Source: CAD feature listing. Evaluate the final solid. Frame: model axes, mm. A direction names the side the tool comes from. Coordinates: 2 decimals unless noted, no trailing zeros. Write each loop counter-clockwise with the first axis right and the second up, starting at its lowest first coordinate (ties: lowest second). Pieces come first, ordered by that corner, then holes. Notation, with made-up numbers: (68, 37.5) - (90, 37.5) arc R7 ccw to (90, 46.5) - close; hole circle Ø4 at (61.25, -19.75). An arc over 180 degrees is marked (long way). One line per question, with ' | ' between items. Start each with the question number.
Q1. Access query for faces 1 (the face through (2.71, -7.95, 20.46)), 2 (the face through (27.035, -3.042, -12.8)), 3 (the face through (0, -10, -26)), 4 (the face through (1.802, -15.437, 5.723)). Directions: +Z, -Z, +X, -X, +Y, -Y. A direction counts if a zero-diameter tool reaches every point of the face in a straight line with its end or side. Return the directions, or none.
Q2. Cut plane D-D, the plane y = -3.5. Return loops of the section in (x, z), plus the area to 3 significant figures.
Q3. Cut plane A-A, the plane y = -15. Return loops of the section in (x, z), plus the area to 3 significant figures.
Q4. Cut plane B-B, the plane z = 0. Return loops of the section in (x, y).
Q5. Cut plane C-C, the plane x = 13.5. Return loops of the section in (y, z), plus the area to 3 significant figures.
Q6. Line query: line 1 (X direction, y = -7.15, z = 0); line 2 (Z direction, x = 3.45, y = -15); line 3 (Z direction, x = 2.2, y = -15). Output: solid intervals per line, ascending.
Q7. Draft query along Y for faces 5 (the face through (2.71, -7.92, -20.64)), 6 (the face through (22.445, -7.507, 0.846)), 7 (the face through (21, 0, -1)), 8 (the face through (8, -20, 0)). Return one class per face: +Y half, -Y half, draft (parallel to the pull), parting line (faces both ways), or undercut.
Q8. Contact query for flat-ended pins moving along their axis: P1, Ø1.5, axis at y = -12, z = 23, coming from the +X side; P2, Ø14.5, axis at x = 16.5, z = -1, coming from the -Y side; P3, Ø6, axis at x = 24, y = -5.5, coming from the -Z side; P4, Ø4, axis at x = 6, z = 22.5, coming from the +Y side. Output: stop coordinate, or through.
```python
from build123d import *

# Parameters (mm, degrees)
SKETCH_1_R          = 6
EXTRUDE_1_DEPTH     = 20
SKETCH_2_R          = 6.1
EXTRUDE_2_DEPTH     = 11
SKETCH_3_R          = 3.4
CUT_EXTRUDE_1_DEPTH = 60.989832472
SKETCH_4_R          = 2.1
CUT_EXTRUDE_2_DEPTH = 10
CUT_EXTRUDE_3_DEPTH = 63.271823484
CUT_EXTRUDE_4_DEPTH = 12
SKETCH_7_R          = 6.5
CUT_EXTRUDE_5_DEPTH = 1
SKETCH_8_R          = 4
CUT_EXTRUDE_6_DEPTH = 60.554848669
CUT_EXTRUDE_7_DEPTH = 60.344586948
CUT_EXTRUDE_8_DEPTH = 2
CHAMFER_1_SIZE      = 0.2


with BuildPart() as part:
    # 草图1 → 凸台-拉伸1 (new body)
    with BuildSketch(Plane(origin=(0, 0, 0), x_dir=(1, 0, 0), z_dir=(0, 1, 0))):
        with BuildLine():
            Line((0, 41.7), (0, 10.918333206))
            ThreePointArc((0, 10.918333206), (-0.463653568, 9.637849063), (-1.63963964, 8.951065962))
            ThreePointArc((-1.63963964, 8.951065962), (-9.1, 0), (-1.63963964, -8.951065962))
            ThreePointArc((-1.63963964, -8.951065962), (-0.463653568, -9.637849063), (0, -10.918333206))
            Line((0, -10.918333206), (0, -41.7))
            ThreePointArc((0, -41.7), (41.7, 0), (0, 41.7))
        make_face()
        with Locations(Location((0, 0, 0), (0, 0, 270))):
            Circle(SKETCH_1_R, mode=Mode.SUBTRACT)
    extrude(amount=EXTRUDE_1_DEPTH)

    # 草图2 → 凸台-拉伸2 (add)
    with BuildSketch(Plane.XZ):
        Circle(SKETCH_2_R)
    extrude(amount=-EXTRUDE_2_DEPTH)

    # 草图3 → 切除-拉伸1 (cut, through all)
    with BuildSketch(Plane(origin=(0, 11, 0), x_dir=(1, 0, 0), z_dir=(0, 1, 0))):
        with Locations(Location((0, 0, 0), (0, 0, 270))):
            Circle(SKETCH_3_R)
    extrude(amount=-CUT_EXTRUDE_1_DEPTH, mode=Mode.SUBTRACT)

    # 草图4 → 切除-拉伸2 (cut)
    with BuildSketch(Plane.ZY):
        with Locations((33.667083302, 15)):
            Circle(SKETCH_4_R)
        with Locations((20.918333206, 10)):
            Circle(SKETCH_4_R)
        with Locations(Location((-33.667083302, 15, 0), (0, 0, 180))):
            Circle(SKETCH_4_R)
        with Locations(Location((-20.918333206, 10, 0), (0, 0, 180))):
            Circle(SKETCH_4_R)
    extrude(amount=-CUT_EXTRUDE_2_DEPTH, mode=Mode.SUBTRACT)


with BuildPart() as body_2:
    # 镜向1: mirrored copy
    add(part.part.mirror(Plane.ZX))

    # 草图5 → 切除-拉伸3 (cut, through all)
    with BuildSketch(Plane(origin=(0, 0, 0), x_dir=(1, 0, 0), z_dir=(0, 1, 0))):
        with BuildLine():
            Line((40.483206395, 10), (40.483206395, -10))
            ThreePointArc((40.483206395, -10), (41.394683878, -5.036878663), (41.7, 0))
            ThreePointArc((41.7, 0), (41.394683878, 5.036878663), (40.483206395, 10))
        make_face()
    extrude(amount=-CUT_EXTRUDE_3_DEPTH, mode=Mode.SUBTRACT)

    # 草图6 → 切除-拉伸4 (cut)
    with BuildSketch(Plane.XZ.offset(20)):
        with BuildLine():
            Line((6, -36.124783736), (6, -6.841783393))
            ThreePointArc((6, -6.841783393), (9.1, 0), (6, 6.841783393))
            Line((6, 6.841783393), (6, 36.124783736))
            ThreePointArc((6, 36.124783736), (6.747974614, 37.684409471), (8.432432432, 38.077474749))
            ThreePointArc((8.432432432, 38.077474749), (39, 0), (8.432432432, -38.077474749))
            ThreePointArc((8.432432432, -38.077474749), (6.747974614, -37.684409471), (6, -36.124783736))
        make_face()
    extrude(amount=-CUT_EXTRUDE_4_DEPTH, mode=Mode.SUBTRACT)

    # 草图7 → 切除-拉伸5 (cut)
    with BuildSketch(Plane.XZ.offset(8)):
        with Locations(Location((16, 0, 0), (0, 0, 270))):
            Circle(SKETCH_7_R)
    extrude(amount=-CUT_EXTRUDE_5_DEPTH, mode=Mode.SUBTRACT)

    # 草图8 → 切除-拉伸6 (cut, through all)
    with BuildSketch(Plane.XZ.offset(7)):
        with Locations(Location((16, 0, 0), (0, 0, 270))):
            Circle(SKETCH_8_R)
    extrude(amount=-CUT_EXTRUDE_6_DEPTH, mode=Mode.SUBTRACT)

    # 草图9 → 切除-拉伸7 (cut, through all)
    with BuildSketch(Plane.XZ.offset(8)):
        with BuildLine():
            ThreePointArc((22.891243611, -20.998113284), (30.339314214, -16.81648203), (35.645345475, -10.122766478))
            ThreePointArc((35.645345475, -10.122766478), (34.525042064, -6.62063566), (31.022911246, -7.740939071))
            ThreePointArc((31.022911246, -7.740939071), (26.965357928, -12.859662729), (21.269774526, -16.057380747))
            ThreePointArc((21.269774526, -16.057380747), (19.6101428, -19.338481558), (22.891243611, -20.998113284))
        make_face()
    extrude(amount=-CUT_EXTRUDE_7_DEPTH, mode=Mode.SUBTRACT)

    # 草图10 → 切除-拉伸8 (cut)
    with BuildSketch(Plane.XZ.offset(8)):
        with BuildLine():
            ThreePointArc((23.712726546, -22.721297552), (31.438040853, -18.105017627), (37.217069697, -11.206224463))
            ThreePointArc((37.217069697, -11.206224463), (35.608500049, -5.048911438), (29.451187024, -6.657481086))
            ThreePointArc((29.451187024, -6.657481086), (25.598501128, -11.256676528), (20.44829159, -14.334196479))
            ThreePointArc((20.44829159, -14.334196479), (17.886958532, -20.159964494), (23.712726546, -22.721297552))
        make_face()
    extrude(amount=-CUT_EXTRUDE_8_DEPTH, mode=Mode.SUBTRACT)

    # 倒角1
    chamfer_1_edges = [body_2.edges().sort_by_distance(p)[0] for p in [
        (0, -10, 41.7),
        (0, -10, -41.7),
    ]]
    chamfer(chamfer_1_edges, length=CHAMFER_1_SIZE)


solid = body_2.part
```
Reply:
1) face 1: -X | face 2: +Y, -Y | face 3: -Z, -X, +Y, -Y | face 4: -Y
2) outline: (-1.64, -8.95) arc R2 cw to (0, -10.92) - (0, -41.5) - (0.2, -41.7) arc R41.7 ccw to (40.48, -10) - (40.48, 10) arc R41.7 ccw to (0.2, 41.7) - (0, 41.5) - (0, 10.92) arc R2 cw to (-1.64, 8.95) arc R9.1 ccw to start; hole circle Ø6.8 at (0, 0); hole circle Ø8 at (16, 0); hole (21.27, -16.06) arc R2.6 ccw to (22.89, -21) arc R22.1 ccw to (35.65, -10.12) arc R2.6 ccw to (31.02, -7.74) arc R16.9 cw to start | area: 2,660 mm^2
3) outline: (-1.64, -8.95) arc R2 cw to (0, -10.92) - (0, -31.57) - (6, -31.57) - (6, -6.84) arc R9.1 ccw to (6, 6.84) - (6, 31.57) - (0, 31.57) - (0, 10.92) arc R2 cw to (-1.64, 8.95) arc R9.1 ccw to start; (0, -41.5) - (0.2, -41.7) arc R41.7 ccw to (40.48, -10) - (40.48, 10) arc R41.7 ccw to (0.2, 41.7) - (0, 41.5) - (0, 35.77) - (6, 35.77) - (6, 36.12) arc R2 cw to (8.43, 38.08) arc R39 cw to (8.43, -38.08) arc R2 cw to (6, -36.12) - (6, -35.77) - (0, -35.77) - close; hole circle Ø12 at (0, 0) | area: 792 mm^2
4) outline: (-9.1, -20) - (-6, -20) - (-6, -11) - (-3.4, -11) - (-3.4, 0) - (-9.1, 0) - close; (3.4, -11) - (6, -11) - (6, -20) - (9.1, -20) - (9.1, -8) - (9.5, -8) - (9.5, -7) - (12, -7) - (12, 0) - (3.4, 0) - close; (20, -7) - (22.5, -7) - (22.5, -8) - (39, -8) - (39, -20) - (40.48, -20) - (40.48, 0) - (20, 0) - close
5) outline: (-20, -39.45) - (0, -39.45) - (0, -3.12) - (-7, -3.12) - (-7, -6) - (-8, -6) - (-8, -36.59) - (-20, -36.59) - close; (-20, 36.59) - (-8, 36.59) - (-8, 6) - (-7, 6) - (-7, 3.12) - (0, 3.12) - (0, 39.45) - (-20, 39.45) - close | area: 644 mm^2
6) line 1: x = -9.1 to -3.4, 3.4 to 9.5, 22.5 to 40.48 | line 2: z = -41.56 to -35.77, -31.57 to -4.91, 4.91 to 31.57, 35.77 to 41.56 | line 3: z = -41.64 to -35.77, -31.57 to -5.58, 5.58 to 31.57, 35.77 to 41.64
7) face 5: undercut | face 6: draft | face 7: +Y half | face 8: -Y half
8) P1: stops at x = 35.27 | P2: stops at y = -8 | P3: stops at z = -36.03 | P4: stops at y = 0
